```python
from build123d import *

# Parameters (mm, degrees)
F1_DEPTH = 20
F4_D     = 8
F4_DEPTH = 30
F4_TIP   = 2.4034424761
F5_D     = 8
F5_DEPTH = 10
F5_TIP   = 2.4034424761


with BuildPart() as f1:
    # F0 (on Right) → F1 (new body)
    with BuildSketch(Plane.YZ):
        Polygon((246.8808323145, 30.0215791241), (246.8808323145, 40.0215791241), (-253.1191676855, 40.0215791241), (-253.1191676855, 30.0215791241), (-246.4204378747, 5.0215791241), (-203.1191676855, -19.9784208759), (196.8808323145, -19.9784208759), (240.1821025037, 5.0215791241), align=None)
    extrude(amount=F1_DEPTH)

    # F4
    with Locations(Plane.XY.offset(40.0215791241)):
        with Locations((11, 186.8808323145), (11, -193.1191676855)):
            Hole(F4_D / 2, depth=F4_DEPTH)
            with Locations((0, 0, -(F4_DEPTH + F4_TIP / 2))):  # 118° drill point
                Cone(0, F4_D / 2, F4_TIP, mode=Mode.SUBTRACT)

    # F5
    with Locations(Plane(origin=(0, 0, 0), x_dir=(0, -1, 0), z_dir=(-1, 0, 0))):
        with Locations((153.1191676855, -10.9784208759), (-146.8808323145, -10.9784208759)):
            Hole(F5_D / 2, depth=F5_DEPTH)
            with Locations((0, 0, -(F5_DEPTH + F5_TIP / 2))):  # 118° drill point
                Cone(0, F5_D / 2, F5_TIP, mode=Mode.SUBTRACT)


solid = f1.part
```
Here's how the part is built. I have some questions about the finished solid (model axes, mm). A direction names the side the tool comes from. Round coordinates to 2 decimals unless told otherwise and drop trailing zeros. Order: outer loops, then holes, each group sorted by start corner. A loop starts at its lowest first (then second) coordinate and runs counter-clockwise, first axis right, second up. Notation, with made-up numbers: M -28.75,86.25 L 19.25,86.25 A27 cw 19.25,118.25 Z; hole C 16.25,-22 d9. An arc over 180 degrees is marked long. Answer as CSV lines item,"result".
Item 1: Please list where these lines run through material, in increasing order: L1, parallel to Y at x = 7.75, z = 34; L2, parallel to Y at x = 6.5, z = -12.5; L3, parallel to X at y = -191, z = 27.5. Write a range as [from, to].
From the geometry:
L1,"[-253.12, -195.45], [-190.79, 184.55], [189.21, 246.88]"
L2,"[-216.07, -156.82], [-149.42, 143.18], [150.58, 209.83]"
L3,"[0, 7.61], [14.39, 20]"
Item 2: For pin 1 (4 mm diameter, centred on x = 5, z = 14.5, fed in from -Y); pin 2 (6 mm diameter, centred on x = 10.5, z = 27, fed in from -Y), each with a flat end and sliding along its axis, tell me the tip position at first contact or that it passes through.
From the geometry:
pin 1,"y = -249.5"
pin 2,"y = -253.11"
Item 3: Which directions (+Z, -Z, +X, -X, +Y, -Y) give clear straight access to the entire face, cutting with the end or side of a thin tool? Please do faces 4 (the cylindrical face through (5.07, -156.07, -8.28)), 5 (the flat face through (10, -6, -19.978)), 6 (the cylindrical face through (11.867, -197.024, 24.812)).
From the geometry:
face 4,"-X"
face 5,"-Z, +X, -X, +Y, -Y"
face 6,"+Z"
Item 4: Imagine slicing it at B-B on z = 15. List the corners of the cut face in (x, y) for me.
From the geometry:
outline,"M 0,-249.09 L 20,-249.09 L 20,242.86 L 0,242.86 Z; hole C 11,-193.12 d8; hole C 11,186.88 d8"
Item 5: Imagine slicing it at A-A on x = 3.5. List the corners of the cut face in (y, z) for me.
From the geometry:
outline,"M -253.12,30.02 L -246.42,5.02 L -203.12,-19.98 L 196.88,-19.98 L 240.18,5.02 L 246.88,30.02 L 246.88,40.02 L -253.12,40.02 Z; hole C -153.12,-10.98 d8; hole C 146.88,-10.98 d8"
Item 6: We'd pull the mould along Y, two halves only. Please class faces 1 (the flat face through (20, -7, 10)), 2 (the flat face through (9.86, 218.228, -7.653)), 3 (the cylindrical face through (11.867, 182.976, 24.812)): +Y half, -Y half, draft (parallel to the pull), parting line (faces both ways), or undercut.
From the geometry:
face 1,"draft"
face 2,"+Y half"
face 3,"undercut"
